Source: CAD feature listing. Evaluate the final solid. Frame: model axes, mm. Coordinates: 2 decimals unless noted, no trailing zeros. Write each loop counter-clockwise with the first axis right and the second up, starting at its lowest first coordinate (ties: lowest second). Pieces come first, ordered by that corner, then holes. Notation, with made-up numbers: (75.25, 48) -> (114.25, 48) arc R19 cw to (114.25, 62) -> close; hole circle Ø11 at (39, 76). An arc over 180 degrees is marked (long way). Write item = value, one per line.
from build123d import *

# Parameters (mm, degrees)
SKETCH1_W           = 190
SKETCH1_H           = 400
SKETCH1_W_2         = 90
SKETCH1_H_2         = 300
BOSS_EXTRUDE1_DEPTH = 25
FILLET1_R           = 25
SKETCH2_R           = 500
BOSS_EXTRUDE2_DEPTH = 1000


with BuildPart() as part:
    # Sketch1 → Boss-Extrude1 (new, symmetric)
    with BuildSketch(Plane.XY):
        with Locations((0, -175)):
            Rectangle(SKETCH1_W, SKETCH1_H)
        with Locations((0, -175)):
            Rectangle(SKETCH1_W_2, SKETCH1_H_2, mode=Mode.SUBTRACT)
    extrude(amount=BOSS_EXTRUDE1_DEPTH, both=True)

    # Fillet1
    fillet1_edges = [part.edges().sort_by_distance(p)[0] for p in [
        (95, -175, 25),
        (0, 25, 25),
        (-45, -175, -25),
        (-45, -25, 0),
        (0, -325, -25),
        (-45, -325, 0),
        (45, -175, -25),
        (45, -325, 0),
        (0, -25, -25),
        (45, -25, 0),
        (-45, -175, 25),
        (0, -325, 25),
        (45, -175, 25),
        (0, -25, 25),
        (-95, -175, 25),
        (0, 25, -25),
        (95, -175, -25),
        (0, -375, -25),
        (-95, -175, -25),
        (0, -375, 25),
        (-95, 25, 0),
        (95, 25, 0),
        (95, -375, 0),
        (-95, -375, 0),
    ]]
    fillet(fillet1_edges, radius=FILLET1_R - 0.0001)  # a hair under: the kernel refuses the full size

    # Sketch2 → Boss-Extrude2 (add)
    with BuildSketch(Plane(origin=(0, -325, 0), x_dir=(1, 0, 0), z_dir=(0, 1, 0))):
        with Locations(Location((0, 0, 0), (0, 0, 270))):
            Circle(SKETCH2_R)
    extrude(amount=-BOSS_EXTRUDE2_DEPTH)


solid = part.part
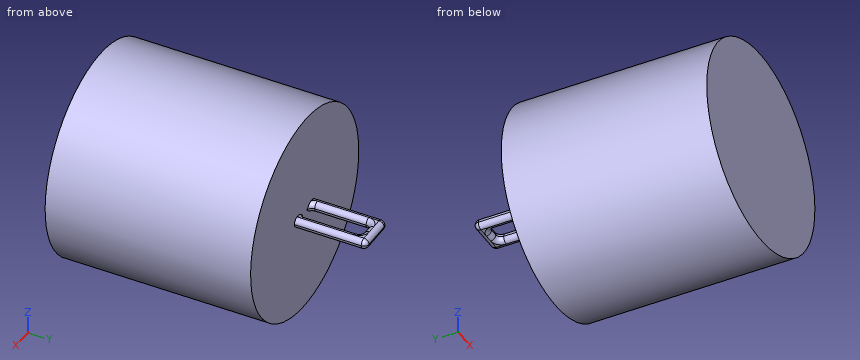
1) First-contact query: pin 1 Ø10 at (x, z) = (-161.5, 371) entering from +Y; pin 2 Ø8 at (x, y) = (-153.5, -775) entering from -Z; pin 3 Ø1.5 at (y, z) = (-937, 191) entering from +X. Flat tips, straight axial feed; report the tip coordinate or a pass-through.
Answer block:
pin_1 = -325
pin_2 = -477.13
pin_3 = 462.39
2) Cut plane D-D, the plane z = -157.5. Output: boundary loops of the cut face in (x, y).
Answer block:
outline = (-474.55, -1325) -> (474.55, -1325) -> (474.55, -325) -> (-474.55, -325) -> close
3) Cut plane C-C, the plane y = -1056. Output: boundary loops of the cut face in (x, z), and give its area (3 significant figures).
Answer block:
outline = circle Ø1000 at (0, 0)
area = 785,000 mm2
4) Material intervals for probe 1 along Y at (x, z) = (-11.5, 135.5); probe 2 along X at (y, z) = (-1130.5, 114); probe 3 along X at (y, z) = (-908, -205.5), sorted ascending. Write a range as [from, to].
Answer block:
probe_1 = [-1325, -325]
probe_2 = [-486.83, 486.83]
probe_3 = [-455.82, 455.82]
